For this review, use the dimensioned drawing (mm, ordinates from the lowest corner) and the shaded views. A direction names the side the tool comes from. Give positions to 0.01 mm unless a question says otherwise; leave off trailing zeros. Write each loop counter-clockwise with the first axis right and the second up, starting at its lowest first coordinate (ties: lowest second). Pieces come first, ordered by that corner, then holes.
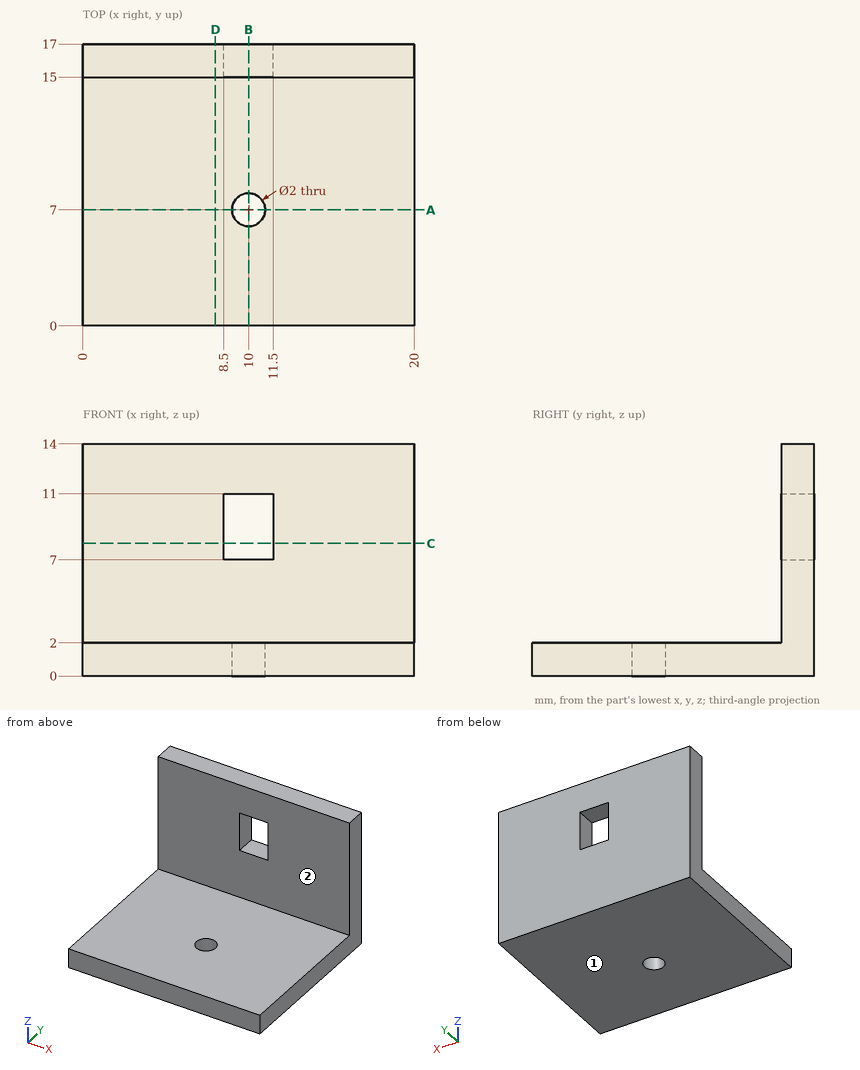
(1) We need section C-C (z = 8). Write out the cut boundary in (x, y).
(2) For L1, parallel to X at y = 7, z = 0.5; L2, parallel to Y at x = 1.75, z = 6.75; L3, parallel to Z at x = 4.25, y = 1.75, list the stretches that pass through material, from the lowest coordinate up.
(3) We need section A-A (y = 7). Write out the cut boundary in (x, z).
(4) We need section B-B (x = 10). Write out the cut boundary in (y, z).
(5) We need section D-D (x = 8). Write out the cut boundary in (y, z).
(6) Tool access review of the marked faces 1 and 2: name each direction out of +Z, -Z, +X, -X, +Y, -Y from which nothing blocks a thin tool from reaching the whole face with its end or side.
(7) Clearance check with flat-ended pins moving along their axes: pin 1 Ø1.2 at (x, y) = (10, 7) entering from +Z; pin 2 Ø2 at (x, y) = (10, 13.5) entering from +Z; pin 3 Ø6 at (x, z) = (7.5, 8.5) entering from -Y. State where each tip first meets the part, or that it passes through.
The answers:
1. outline: (0, 15) - (8.5, 15) - (8.5, 17) - (0, 17) - close; (11.5, 15) - (20, 15) - (20, 17) - (11.5, 17) - close
2. L1: x = 0 to 9, 11 to 20
2. L2: y = 15 to 17
2. L3: z = 0 to 2
3. outline: (0, 0) - (9, 0) - (9, 2) - (0, 2) - close; (11, 0) - (20, 0) - (20, 2) - (11, 2) - close
4. outline: (0, 0) - (6, 0) - (6, 2) - (0, 2) - close; (8, 0) - (17, 0) - (17, 7) - (15, 7) - (15, 2) - (8, 2) - close; (15, 11) - (17, 11) - (17, 14) - (15, 14) - close
5. outline: (0, 0) - (17, 0) - (17, 14) - (15, 14) - (15, 2) - (0, 2) - close
6. face 1: -Z, +X, -X, +Y, -Y
6. face 2: +Z, +X, -X, -Y
7. pin 1: passes through
7. pin 2: stops at z = 2
7. pin 3: stops at y = 15
